from build123d import *

# Parameters (mm, degrees)
POCKET003_DEPTH         = 0.5
POLARPATTERN_COUNT      = 6
BODY003_PLACEMENT_ANGLE = 180


with BuildPart() as part:
    # Sketch022 → Revolution003 (revolve)
    with BuildSketch(Plane.YZ):
        Polygon((16, 0), (18, 0), (18, 1.25), (17.75, 1.5), (16, 1.5), align=None)
    revolve(axis=Axis((0, 0, 0), (0, 0, 1)))

    # Sketch023 (on Face4 of Revolution003) → Pocket003 (cut)
    with BuildSketch(Plane(origin=(0, 0, 1.5), x_dir=(0, -1, 0), z_dir=(0, 0, 1))):
        with BuildLine():
            Line((-0.75, 15.982412), (-0.75, 17.482412))
            ThreePointArc((0.75, 17.482412), (0, 17.498492), (-0.75, 17.482412))
            Line((0.75, 15.982412), (0.75, 17.482412))
            Line((-0.75, 15.982412), (0.75, 15.982412))
        make_face()
    pocket003 = extrude(amount=-POCKET003_DEPTH, mode=Mode.SUBTRACT)

    # PolarPattern: Pocket003 ×6 about axis
    polarpattern_axis = Axis((0, 0, 1.5), (0, 0, 1))
    for i in range(1, POLARPATTERN_COUNT):
        add(pocket003.rotate(polarpattern_axis, i * 360 / POLARPATTERN_COUNT), mode=Mode.SUBTRACT)


with BuildPart() as part_1:
    # Body003 placement: moved
    add(part.part.moved(Location((0, 0, 0))).rotate(Axis((0, 0, 0), (1, 0, 0)), BODY003_PLACEMENT_ANGLE))


solid = part_1.part
Check sheet for the modelled part. Datum: model origin and axes. Units: mm. A direction names the side the tool comes from. Give positions to 0.01 mm unless a question says otherwise; leave off trailing zeros. Loops run counter-clockwise (first coordinate to the right, second up) from the corner with the lowest first, then second, coordinate; pieces in that order, holes last. Notation, with made-up numbers: M 18,20.5 L 77,20.5 A31 cw 77,49.5 Z; hole C 6,-4.5 d10. An arc over 180 degrees is marked long. Return JSON: item names as keys, results as strings. Group by question number.
1. Thickness scan on L1, parallel to Y at x = 0, z = -0.55; L2, parallel to Y at x = 9, z = -1.15. Record the ranges inside material, lowest first.
2. Cross-section at B-B on y = 0. Record the boundary of the cut face in (x, z), plus the area to 3 significant figures.
3. Mould release check, pull along Y, two halves, no side actions. Record for faces 3 (the cylindrical face through (-17.847, 2.343, -0.634)), 4 (the flat face through (11, -12, 0)), 5 (the flat face through (-8, -15, -1)): released by +Y, released by -Y, zero draft, split by the parting line, or undercut.
4. Go/stop test with a flat-tipped pin: pin 1 (0.5 mm diameter, centred on x = -16.5, y = 0, fed in from -Z). Record where the tip stops, or that it passes through.
5. Tool access check on faces 1 (the flat face through (17, 0, -1)), 2 (the cylindrical face through (15.62, 3.47, -0.74)). Record the directions out of +Z, -Z, +X, -X, +Y, -Y that give a thin tool (end or side, any length) a straight path to the whole face; none if there is none.
6. Cross-section at C-C on z = -0.6. Record the boundary of the cut face in (x, y).
7. Cross-section at A-A on x = 0. Record the boundary of the cut face in (y, z).
Return value:
{
 "1": {"L1": "-18 to -16, 16 to 18", "L2": "-15.59 to -15.01, -14.09 to -13.23, 13.23 to 14.09, 15.01 to 15.59"},
 "2": {"outline": "M -18,-1.25 L -17.75,-1.5 L -17.5,-1.5 L -17.5,-1 L -16,-1 L -16,0 L -18,0 Z; M 16,-1 L 17.5,-1 L 17.5,-1.5 L 17.75,-1.5 L 18,-1.25 L 18,0 L 16,0 Z", "area": "4.44 mm^2"},
 "3": {"face 3": "split by the parting line", "face 4": "zero draft", "face 5": "undercut"},
 "4": {"pin 1": "z = -1"},
 "5": {"face 1": "-Z", "face 2": "+Z, -Z"},
 "6": {"outline": "C 0,0 d36; hole C 0,0 d32"},
 "7": {"outline": "M -18,-1.25 L -17.75,-1.5 L -16,-1.5 L -16,0 L -18,0 Z; M 16,-1.5 L 17.75,-1.5 L 18,-1.25 L 18,0 L 16,0 Z"}
}
